Geometry: final body of the model. Coordinates: model frame, mm. A direction names the side the tool comes from. Give positions to 0.01 mm unless a question says otherwise; leave off trailing zeros. Loops run counter-clockwise (first coordinate to the right, second up) from the corner with the lowest first, then second, coordinate; pieces in that order, holes last.
```python
from build123d import *

# Parameters (mm, degrees)
F0_W     = 63.5
F0_H     = 42
F0_R     = 2
F0_R_2   = 11.5
F1_DEPTH = 4
F2_SIZE  = 4
F3_W     = 13
F3_H     = 3
F4_DEPTH = 30
F5_R     = 5
F6_R     = 4
F7_R     = 2.5
F7_R_2   = 1.75
F8_DEPTH = 3


with BuildPart() as f1:
    # F0 (on Front) → F1 (new body)
    with BuildSketch(Plane.XZ):
        with Locations((11.25, -0.25)):
            Rectangle(F0_W, F0_H)
        with Locations((-15.25, -16)):
            Circle(F0_R, mode=Mode.SUBTRACT)
        with Locations((15.75, -16)):
            Circle(F0_R, mode=Mode.SUBTRACT)
        Circle(F0_R_2, mode=Mode.SUBTRACT)
        with Locations((-15.25, 15.5)):
            Circle(F0_R, mode=Mode.SUBTRACT)
        with Locations((15.75, 15.5)):
            Circle(F0_R, mode=Mode.SUBTRACT)
    extrude(amount=F1_DEPTH)

    # F2
    f2_edges = [f1.edges().sort_by_distance(p)[0] for p in [
        (-20.5, -2, -21.25),
        (-20.5, -2, 20.75),
    ]]
    chamfer(f2_edges, length=F2_SIZE)

    # F3 (on face) → F4 (join)
    with BuildSketch(Plane.XZ.offset(4)):
        with Locations((33.5, -5.75)):
            Rectangle(F3_W, F3_H)
    extrude(amount=F4_DEPTH)

    # F5
    f5_edges = [f1.edges().sort_by_distance(p)[0] for p in [
        (40, -34, -5.75),
        (27, -34, -5.75),
    ]]
    fillet(f5_edges, radius=F5_R)

    # F6
    f6_edges = [f1.edges().sort_by_distance(p)[0] for p in [
        (43, -2, 20.75),
        (43, -2, -21.25),
    ]]
    fillet(f6_edges, radius=F6_R)

    # F7 (on face) → F8 (cut, through all)
    with BuildSketch(Plane.XY.offset(-4.25)):
        with Locations((33.5, -21.5)):
            Circle(F7_R)
        with Locations((33.5, -30.5)):
            Circle(F7_R_2)
        with Locations((33.5, -12.5)):
            Circle(F7_R_2)
    extrude(amount=-F8_DEPTH, mode=Mode.SUBTRACT)


solid = f1.part
```
Q1. Section query D-D, the plane x = 33.5. Return loops of the section in (y, z), and give its area (3 significant figures).
Q2. Material intervals for probe 1 along Y at (x, z) = (33.5, -5.15); probe 2 along Z at (x, y) = (0, -2.95); probe 3 along Y at (x, z) = (33, -6), sorted ascending.
Q3. Section query A-A, the plane z = 0. Return loops of the section in (x, y), and give its area (3 significant figures).
Q4. Section query C-C, the plane z = 15.5. Return loops of the section in (x, y), and give its area (3 significant figures).
Q5. Section query B-B, the plane x = 15.75. Return loops of the section in (y, z).
Q6. Pin query (flat end, axial travel): pin 1 Ø14.5 at (x, y) = (31, -17) entering from +Z; pin 2 Ø3.5 at (y, z) = (-13.5, -5.5) entering from +X; pin 3 Ø5 at (x, z) = (24.5, -11) entering from -Y. Return the tip coordinate at first contact, or that it passes through.
Q7. Mould query, pull axis X, two halves, no side actions, for faces 5 (the face through (-18.47, -1.97, 18.78)), 6 (the face through (-1.5, -2, 11.4)), 7 (the face through (11, -2, -21.25)), 8 (the face through (-15.51, -1.972, 17.483)). Classes: +X half, -X half, draft (parallel to the pull), parting line (faces both ways), or undercut.
Q8. Reachability of faces 1 (the face through (40, -16, -6)), 2 (the face through (33.4, -18.8, -4.25)), 3 (the face through (27, -16, -6)), 4 (the face through (33.4, -18.8, -7.25)) from +Z, -Z, +X, -X, +Y, -Y: full face, straight path, thin tool, end or side. Return the list, or none.
Resolved:
1. outline: (-34, -7.25) - (-32.25, -7.25) - (-32.25, -4.25) - (-34, -4.25) - close; (-28.75, -7.25) - (-24, -7.25) - (-24, -4.25) - (-28.75, -4.25) - close; (-19, -7.25) - (-14.25, -7.25) - (-14.25, -4.25) - (-19, -4.25) - close; (-10.75, -7.25) - (-4, -7.25) - (-4, -21.25) - (0, -21.25) - (0, 20.75) - (-4, 20.75) - (-4, -4.25) - (-10.75, -4.25) - close
1. area: 222 mm2
2. probe 1: y = -34 to -32.25, -28.75 to -24, -19 to -14.25, -10.75 to 0
2. probe 2: z = -21.25 to -11.5, 11.5 to 20.75
2. probe 3: y = -34 to -32.18, -28.82 to -23.95, -19.05 to -14.18, -10.82 to 0
3. outline: (-20.5, -4) - (-11.5, -4) - (-11.5, 0) - (-20.5, 0) - close; (11.5, -4) - (43, -4) - (43, 0) - (11.5, 0) - close
3. area: 162 mm2
4. outline: (-20.5, -4) - (-17.25, -4) - (-17.25, 0) - (-20.5, 0) - close; (-13.25, -4) - (13.75, -4) - (13.75, 0) - (-13.25, 0) - close; (17.75, -4) - (43, -4) - (43, 0) - (17.75, 0) - close
4. area: 222 mm2
5. outline: (-4, -21.25) - (0, -21.25) - (0, -18) - (-4, -18) - close; (-4, -14) - (0, -14) - (0, 13.5) - (-4, 13.5) - close; (-4, 17.5) - (0, 17.5) - (0, 20.75) - (-4, 20.75) - close
6. pin 1: stops at z = -4.25
6. pin 2: stops at x = 40
6. pin 3: stops at y = -4
7. face 5: -X half
7. face 6: undercut
7. face 7: draft
7. face 8: undercut
8. face 1: +Z, -Z, +X, -Y
8. face 2: +Z, +X, -X, -Y
8. face 3: +Z, -Z, -X, -Y
8. face 4: -Z, +X, -X, -Y
